For this review, take the finished solid that the model builds, in its own axes (mm). A direction names the side the tool comes from. Round coordinates to 2 decimals unless told otherwise and drop trailing zeros. Loops run counter-clockwise (first coordinate to the right, second up) from the corner with the lowest first, then second, coordinate; pieces in that order, holes last.
1) Wall thickness on L1, parallel to X at y = 4.5, z = -12.7; L2, parallel to X at y = 4.75, z = -21; L3, parallel to X at y = 2.75, z = -12.7: over which ranges is each line inside the solid? List them lowest first.
2) Insertion check: pin 1 (5 mm diameter, centred on x = 48, z = -17, fed in from +Y). The pin has a flat end and moves straight along its axis. Give the tip position at first contact, or say it passes through.
3) Take a section at A-A (y = 5.75). State the section outline as (x, z) points.
4) Mouldability with a two-part tool opening along X and no side actions: class faces 1 (the flat face through (0, 3, -13)), 2 (the cylindrical face through (5.54, 3.131, -11.666)), 3 (the flat face through (33, 0, -13)) as pulls with the +X half, pulls with the -X half, needs draft (parallel to the pull), parting line crosses it, or undercut.
5) Take a section at B-B (z = -12.7). State the section outline as (x, y) points.
6) Tool access review of faces 4 (the flat face through (66.04, 3, -13)), 5 (the flat face through (48, 3.81, -13)): name each direction out of +Z, -Z, +X, -X, +Y, -Y from which nothing blocks a thin tool from reaching the whole face with its end or side.
7) Take a section at C-C (z = -9.75). State the section outline as (x, y) points.
8) Take a section at D-D (x = 17.5). State the section outline as (y, z) points, then the cut area to 3 significant figures.
```python
from build123d import *

# Parameters (mm, degrees)
SKETCH1_W            = 66.04
SKETCH1_H            = 25.4
BOSS_EXTRUDE1_DEPTH  = 6.35
M3_CLEARANCE_HOLE1_D = 3.4
SKETCH5_W            = 6.35
SKETCH5_H            = 2.54
CUT_EXTRUDE1_DEPTH   = 72.040580656


with BuildPart() as part:
    # Sketch1 → Boss-Extrude1 (new body)
    with BuildSketch(Plane(origin=(0, 0, 0), x_dir=(1, 0, 0), z_dir=(0, 1, 0))):
        with Locations((33.02, 12.7)):
            Rectangle(SKETCH1_W, SKETCH1_H)
    extrude(amount=BOSS_EXTRUDE1_DEPTH)

    # M3 Clearance Hole1 (through all)
    with Locations(Plane(origin=(0, 6.35, 0), x_dir=(1, 0, 0), z_dir=(0, 1, 0))):
        with Locations((4.191, 12.7), (61.849, 12.7)):
            Hole(M3_CLEARANCE_HOLE1_D / 2)

    # Sketch5 → Cut-Extrude1 (cut, through all)
    with BuildSketch(Plane.XY):
        with Locations((48.133, 5.08)):
            Rectangle(SKETCH5_W, SKETCH5_H)
        with Locations((17.907, 5.08)):
            Rectangle(SKETCH5_W, SKETCH5_H)
    extrude(amount=-CUT_EXTRUDE1_DEPTH, mode=Mode.SUBTRACT)


solid = part.part
```
Response:
1. L1: x = 0 to 2.49, 5.89 to 14.73, 21.08 to 44.96, 51.31 to 60.15, 63.55 to 66.04
1. L2: x = 0 to 14.73, 21.08 to 44.96, 51.31 to 66.04
1. L3: x = 0 to 2.49, 5.89 to 60.15, 63.55 to 66.04
2. pin 1: stops at y = 3.81
3. outline: (0, -25.4) - (14.73, -25.4) - (14.73, 0) - (0, 0) - close; (21.08, -25.4) - (44.96, -25.4) - (44.96, 0) - (21.08, 0) - close; (51.31, -25.4) - (66.04, -25.4) - (66.04, 0) - (51.31, 0) - close; hole circle Ø3.4 at (4.19, -12.7); hole circle Ø3.4 at (61.85, -12.7)
4. face 1: pulls with the -X half
4. face 2: undercut
4. face 3: needs draft
5. outline: (0, 0) - (2.49, 0) - (2.49, 6.35) - (0, 6.35) - close; (5.89, 0) - (60.15, 0) - (60.15, 6.35) - (51.31, 6.35) - (51.31, 3.81) - (44.96, 3.81) - (44.96, 6.35) - (21.08, 6.35) - (21.08, 3.81) - (14.73, 3.81) - (14.73, 6.35) - (5.89, 6.35) - close; (63.55, 0) - (66.04, 0) - (66.04, 6.35) - (63.55, 6.35) - close
6. face 4: +Z, -Z, +X, +Y, -Y
6. face 5: +Z, -Z, +Y
7. outline: (0, 0) - (66.04, 0) - (66.04, 6.35) - (51.31, 6.35) - (51.31, 3.81) - (44.96, 3.81) - (44.96, 6.35) - (21.08, 6.35) - (21.08, 3.81) - (14.73, 3.81) - (14.73, 6.35) - (0, 6.35) - close
8. outline: (0, -25.4) - (3.81, -25.4) - (3.81, 0) - (0, 0) - close
8. area: 96.8 mm2
